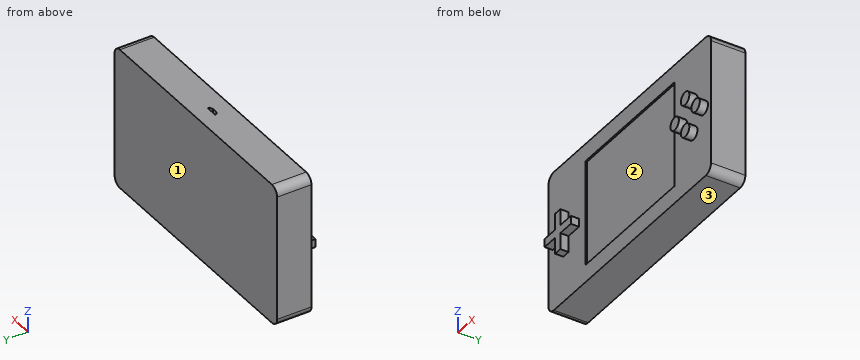
from build123d import *

# Parameters (mm, degrees)
F1_DEPTH = 21
F4_DEPTH = 5
F5_R     = 4
F6_DEPTH = 5
F2_W     = 85
F2_H     = 65
F7_DEPTH = 1
F9_DEPTH = 11


with BuildPart() as f1:
    # F0 (on Front) → F1 (new body)
    with BuildSketch(Plane.XZ):
        with BuildLine():
            Line((-72.5, -43.25), (72.5, -43.25))
            ThreePointArc((72.5, -43.25), (76.035534, -41.785534), (77.5, -38.25))
            Line((77.5, -38.25), (77.5, 38.25))
            ThreePointArc((77.5, 38.25), (76.035534, 41.785534), (72.5, 43.25))
            Line((72.5, 43.25), (-72.5, 43.25))
            ThreePointArc((-72.5, 43.25), (-76.035534, 41.785534), (-77.5, 38.25))
            Line((-77.5, 38.25), (-77.5, -38.25))
            ThreePointArc((-77.5, -38.25), (-76.035534, -41.785534), (-72.5, -43.25))
        make_face()
    extrude(amount=-F1_DEPTH)

    # F3 (on face) → F4 (join)
    with BuildSketch(Plane.XZ):
        Polygon((-48.470394, -5), (-48.470394, 0), (-58.470394, 0), (-58.470394, 10), (-63.470394, 10), (-63.470394, 0), (-73.470394, 0), (-73.470394, -5), (-63.470394, -5), (-63.470394, -15), (-58.470394, -15), (-58.470394, -5), align=None)
    extrude(amount=F4_DEPTH)

    # F5 (on Front) → F6 (join)
    with BuildSketch(Plane.XZ):
        with Locations((60.575662, 10)):
            Circle(F5_R)
        with Locations((70.575662, 0)):
            Circle(F5_R)
        with Locations((60.575662, -10)):
            Circle(F5_R)
        with Locations((50.575662, 0)):
            Circle(F5_R)
    extrude(amount=F6_DEPTH)

    # F2 (on face) → F7 (cut)
    with BuildSketch(Plane.XZ):
        Rectangle(F2_W, F2_H)
    extrude(amount=-F7_DEPTH, mode=Mode.SUBTRACT)

    # F8 (on face) → F9 (cut)
    with BuildSketch(Plane.XY.offset(43.25)):
        Polygon((-1.676761, 9.575), (1.676761, 9.575), (3.45, 10.5), (3.45, 11.425), (-3.45, 11.425), (-3.45, 10.5), align=None)
    extrude(amount=-F9_DEPTH, mode=Mode.SUBTRACT)


solid = f1.part
Work out the finished part from the listing and answer in its coordinate system (mm). Face numbers are marked on the shaded views. Give positions to 0.01 mm unless a question says otherwise; leave off trailing zeros. Loops run counter-clockwise (first coordinate to the right, second up) from the corner with the lowest first, then second, coordinate; pieces in that order, holes last. Notation, with made-up numbers: (-19, -26) -> (25, -26) arc R13 ccw to (25, -3) -> close; hole circle Ø10 at (60, 68.5). An arc over 180 degrees is marked (long way). Use a Markdown table: item, result. Add a question column.
1. Determine the mould class of the marked faces 1, 2 and 3 for opening direction Z: released by +Z, released by -Z, zero draft, split by the parting line, or undercut.
2. Section A-A on z = -10 is taken. Determine the outline of the cut face in (x, y), and give its area (4 significant figures).
3. Section D-D on x = 61 is taken. Determine the outline of the cut face in (y, z).
4. Section B-B on x = -9 is taken. Determine the outline of the cut face in (y, z), and give its area (3 significant figures).
5. Flat-ended cylindrical pins translate along their axes: pin 1 Ø4 at (y, z) = (-3, -2) entering from +X; pin 2 Ø2 at (x, z) = (1, 38) entering from -Y; pin 3 Ø2.5 at (x, y) = (-55, -3) entering from -Z. Find the tip coordinate at first contact, or state that the pin passes through.
6. Section C-C on z = 15.5 is taken. Determine the outline of the cut face in (x, y).
7. Find the intervals of material crossed by probe 1 along Y at (x, z) = (-63.5, 28); probe 2 along Y at (x, z) = (17, -31.5); probe 3 along X at (y, z) = (-2.5, -13), in increasing order.
Results below:
| question | item | result |
|---|---|---|
| 1 | face 1 | zero draft |
| 1 | face 2 | undercut |
| 1 | face 3 | released by -Z |
| 2 | outline | (-77.5, 0) -> (-63.47, 0) -> (-63.47, -5) -> (-58.47, -5) -> (-58.47, 0) -> (-42.5, 0) -> (-42.5, 1) -> (42.5, 1) -> (42.5, 0) -> (56.58, 0) -> (56.58, -5) -> (64.58, -5) -> (64.58, 0) -> (77.5, 0) -> (77.5, 21) -> (-77.5, 21) -> close |
| 2 | area | 3,235 mm^2 |
| 3 | outline | (-5, -13.98) -> (0, -13.98) -> (0, -43.25) -> (21, -43.25) -> (21, 43.25) -> (0, 43.25) -> (0, 13.98) -> (-5, 13.98) -> (-5, 6.02) -> (0, 6.02) -> (0, -6.02) -> (-5, -6.02) -> close |
| 4 | outline | (0, -43.25) -> (21, -43.25) -> (21, 43.25) -> (0, 43.25) -> (0, 32.5) -> (1, 32.5) -> (1, -32.5) -> (0, -32.5) -> close |
| 4 | area | 1,750 mm^2 |
| 5 | pin 1 | stops at x = 74.58 |
| 5 | pin 2 | stops at y = 0 |
| 5 | pin 3 | stops at z = -5 |
| 6 | outline | (-77.5, 0) -> (-42.5, 0) -> (-42.5, 1) -> (42.5, 1) -> (42.5, 0) -> (77.5, 0) -> (77.5, 21) -> (-77.5, 21) -> close |
| 7 | probe 1 | y = 0 to 21 |
| 7 | probe 2 | y = 1 to 21 |
| 7 | probe 3 | x = -63.47 to -58.47, 57.93 to 63.22 |
